Here's how the part is built. I have some questions about the finished solid (model axes, mm). A direction names the side the tool comes from. Coordinates: 2 decimals unless noted, no trailing zeros. Use one line per item in the form item = value. Start each with the question number.
1. I want a section at A-A, the plane x = 0. Count the separate pieces of the cut face and the enclosed holes in it, plus the area to 3 significant figures.
2. On a 3-axis mill with a long thin cutter (end or side, diameter ignored), from which of +Z, -Z, +X, -X, +Y, -Y can I reach the whole of each face in a straight line? I mean faces 1 (the face through (14.224, -7, 6)), 2 (the face through (31.83, 44.77, -29.18)), 3 (the face through (7.501, -19.734, 14.422)). Say none if no direction works.
3. I'm going to push flat-ended pins straight in: pin 1 Ø8.5 at (x, y) = (-6.5, 5.5) entering from -Z; pin 2 Ø2 at (y, z) = (24.5, 26) entering from -X; pin 3 Ø20 at (x, y) = (0, 0) entering from +Z; pin 4 Ø10 at (x, z) = (17, -39) entering from +Y. Where does each tip first touch, or does it pass through?
4. Please list where these lines run through material, in increasing order: line 1 along X through (y, z) = (-1, 21.5); line 2 along X through (y, z) = (0, -9). Write a range as [from, to].
5. Thinking about a two-plate mould opening in Z: for faces 4 (the face through (-25.4, 12, -12)), 5 (the face through (44, 50.8, 1)), 6 (the face through (31, 0, -35.56)), which applies, released by +Z, released by -Z, zero draft, split by the parting line, or undercut?
from build123d import *

# Parameters (mm, degrees)
F0_W          = 101.6
F0_H          = 101.6
F1_DEPTH      = 50.8
F1_DEPTH_BACK = 50.8


with BuildPart() as f1:
    # F0 (on Top) → F1 (new body, two sides)
    with BuildSketch(Plane.XY) as f1_sk:
        Rectangle(F0_W, F0_H)
    extrude(amount=F1_DEPTH)
    extrude(f1_sk.sketch, amount=-F1_DEPTH_BACK)

    # F2 (on Top) → F3 (revolve, cut)
    with BuildSketch(Plane.XY):
        Polygon((0, 50.8), (-41.1113, 50.8), (-43.18, 50.8), (-43.18, 35.56), (-30.48, 35.56), (-30.48, 25.4), (-16.256, 25.4), (-16.256, 14.224), (-7.62, 14.224), (-7.62, 0), (0, 0), align=None)
    revolve(axis=Axis((0, 25.4, 0), (0, -1, 0)), mode=Mode.SUBTRACT)

    # F4 (on Top) → F5 (revolve, cut)
    with BuildSketch(Plane.XY):
        Polygon((0, -50.8), (13.884519, -50.8), (43.18, -50.8), (43.18, -35.56), (30.48, -35.56), (30.48, -25.4), (16.256, -25.4), (16.256, -14.224), (7.62, -14.224), (7.62, 0), (0, 0), align=None)
    revolve(axis=Axis((0, -25.4, 0), (0, 1, 0)), mode=Mode.SUBTRACT)

    # F6 (on Top) → F7 (revolve, cut)
    with BuildSketch(Plane.XY):
        Polygon((50.8, 0), (50.8, 16.378657), (50.8, 43.18), (35.56, 43.18), (35.56, 30.48), (25.4, 30.48), (25.4, 16.256), (14.224, 16.256), (14.224, 7.62), (0, 7.62), (0, 0), align=None)
    revolve(axis=Axis((25.4, 0, 0), (-1, 0, 0)), mode=Mode.SUBTRACT)

    # F8 (on Top) → F9 (revolve, cut)
    with BuildSketch(Plane.XY):
        Polygon((-50.8, 0), (-50.8, -43.18), (-35.56, -43.18), (-35.56, -30.48), (-25.4, -30.48), (-25.4, -16.256), (-14.224, -16.256), (-14.224, -7.62), (0, -7.62), (0, 0), align=None)
    revolve(axis=Axis((-25.4, 0, 0), (1, 0, 0)), mode=Mode.SUBTRACT)

    # F10 (on Right) → F11 (revolve, cut)
    with BuildSketch(Plane.YZ):
        Polygon((-7.62, 0), (0, 0), (0, 50.8), (-43.18, 50.8), (-43.18, 35.56), (-30.48, 35.56), (-30.48, 25.4), (-16.256, 25.4), (-16.256, 14.224), (-7.62, 14.224), align=None)
    revolve(axis=Axis((0, 0, 25.4), (0, 0, -1)), mode=Mode.SUBTRACT)

    # F12 (on Right) → F13 (revolve, cut)
    with BuildSketch(Plane.YZ):
        Polygon((7.62, 0), (0, 0), (0, -50.8), (43.18, -50.8), (43.18, -35.56), (30.48, -35.56), (30.48, -25.4), (16.256, -25.4), (16.256, -14.224), (7.62, -14.224), align=None)
    revolve(axis=Axis((0, 0, -25.4), (0, 0, 1)), mode=Mode.SUBTRACT)


solid = f1.part
Answer list:
q1.separate_pieces = 16
q1.enclosed_holes = 0
q1.area = 844 mm²
q2.face_1 = +X
q2.face_2 = +Y
q2.face_3 = -Y
q3.pin_1 = -14.22
q3.pin_2 = -35.56
q3.pin_3 = 14.22
q3.pin_4 = 50.8
q4.line_1 = [-25.4, -16.23], [16.23, 25.4]
q4.line_2 = [-14.22, -7.62], [7.62, 14.22]
q5.face_4 = undercut
q5.face_5 = zero draft
q5.face_6 = released by -Z
